Input: part model. Units: mm. Frame: model coordinates. Face numbers are marked on the shaded views. A direction names the side the tool comes from. Give positions to 0.01 mm unless a question says otherwise; leave off trailing zeros. Loops run counter-clockwise (first coordinate to the right, second up) from the corner with the lowest first, then second, coordinate; pieces in that order, holes last. Notation, with made-up numbers: (56, 54) - (87, 54) arc R18 ccw to (87, 76) - close; hole circle Ø8 at (-11, 7). An arc over 180 degrees is marked (long way). Answer as a JSON object with one key per item and string values. Group by question number.
(1) Section query D-D (x = 24.13). Return loops of the section in (y, z).
(2) Section query B-B (z = -5.08). Return loops of the section in (x, y).
(3) Mould query, pull axis Z, two halves, no side actions, for the marked faces 3, 4, 5 and 6. Classes: +Z half, -Z half, draft (parallel to the pull), parting line (faces both ways), or undercut.
(4) Section query C-C (y = 16.5). Return loops of the section in (x, z), plus the area to 3 significant figures.
(5) Section query A-A (x = 5.08). Return loops of the section in (y, z).
(6) Material intervals for L1, parallel to Z at x = 5.08, y = 2.9; L2, parallel to X at y = 2.55, z = -5.08; L3, parallel to Z at x = 24.13, y = 2.15, sorted ascending.
(7) Pin query (flat end, axial travel): P1, Ø1, axis at y = 6, z = -3, coming from the +X side; P2, Ø12, axis at y = 25, z = -22.5, coming from the -X side; P3, Ø9.5, axis at y = 23, z = -16, coming from the +X side; P4, Ø6, axis at x = 14.5, y = 25, coming from the +Z side. Return the tip coordinate at first contact, or that it passes through.
(8) Access query for the marked faces 1 and 2. Directions: +Z, -Z, +X, -X, +Y, -Y. A direction counts if a zero-diameter tool reaches every point of the face in a straight line with its end or side. Return the directions, or none.
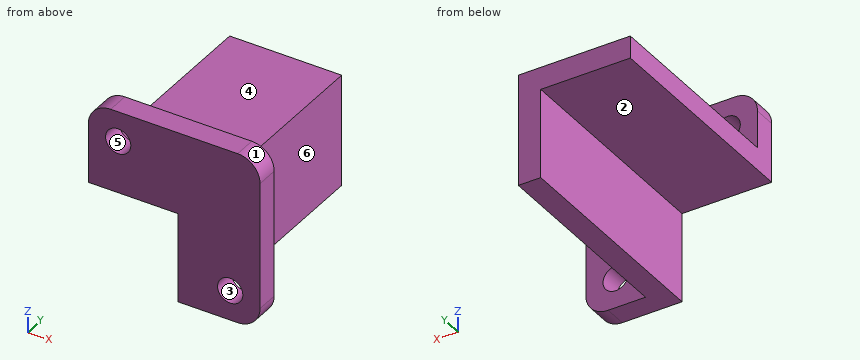
```python
from build123d import *

# Parameters (mm, degrees)
BOSS_EXTRUDE1_DEPTH = 3.81
BOSS_EXTRUDE2_DEPTH = 34.29
SKETCH3_R           = 2.15
CUT_EXTRUDE1_DEPTH  = 4.81
FILLET1_R           = 3.81


with BuildPart() as part:
    # Sketch1 → Boss-Extrude1 (new body)
    with BuildSketch(Plane(origin=(0, 0, 0), x_dir=(1, 0, 0), z_dir=(0, 1, 0))):
        Polygon((29.21, 0), (29.21, 29.21), (15.24, 29.21), (15.24, 13.97), (0, 13.97), (0, 0), align=None)
    extrude(amount=BOSS_EXTRUDE1_DEPTH)

    # Sketch2 → Boss-Extrude2 (add)
    with BuildSketch(Plane(origin=(0, 3.81, 0), x_dir=(1, 0, 0), z_dir=(0, 1, 0))):
        Polygon((0, 13.97), (15.24, 13.97), (15.24, 29.21), (19.05, 29.21), (19.05, 10.16), (0, 10.16), align=None)
    extrude(amount=BOSS_EXTRUDE2_DEPTH)

    # Sketch3 → Cut-Extrude1 (cut, through all)
    with BuildSketch(Plane(origin=(0, 3.81, 0), x_dir=(1, 0, 0), z_dir=(0, 1, 0))):
        with Locations((5.08, 5.08)):
            Circle(SKETCH3_R)
        with Locations((24.13, 24.13)):
            Circle(SKETCH3_R)
    extrude(amount=-CUT_EXTRUDE1_DEPTH, mode=Mode.SUBTRACT)

    # Fillet1
    fillet1_edges = [part.edges().sort_by_distance(p)[0] for p in [
        (29.21, 1.905, -29.21),
        (29.21, 1.905, 0),
        (0, 1.905, 0),
    ]]
    fillet(fillet1_edges, radius=FILLET1_R)


solid = part.part
```
Recorded:
{
 "1": {"outline": "(0, -29.21) - (3.81, -29.21) - (3.81, -26.28) - (0, -26.28) - close; (0, -21.98) - (3.81, -21.98) - (3.81, 0) - (0, 0) - close"},
 "2": {"outline": "(0, 0) - (2.93, 0) - (2.93, 3.81) - (0, 3.81) - close; (7.23, 0) - (29.21, 0) - (29.21, 3.81) - (7.23, 3.81) - close"},
 "3": {"face 3": "undercut", "face 4": "+Z half", "face 5": "undercut", "face 6": "draft"},
 "4": {"outline": "(0, -13.97) - (15.24, -13.97) - (15.24, -29.21) - (19.05, -29.21) - (19.05, -10.16) - (0, -10.16) - close", "area": "131 mm^2"},
 "5": {"outline": "(0, -13.97) - (38.1, -13.97) - (38.1, -10.16) - (3.81, -10.16) - (3.81, -7.23) - (0, -7.23) - close; (0, -2.93) - (3.81, -2.93) - (3.81, 0) - (0, 0) - close"},
 "6": {"L1": "z = -13.97 to -7.23, -2.93 to 0", "L2": "x = 0 to 2.93, 7.23 to 29.21", "L3": "z = -29.21 to -26.28, -21.98 to 0"},
 "7": {"P1": "passes through", "P2": "stops at x = 15.24", "P3": "stops at x = 19.05", "P4": "stops at z = -10.16"},
 "8": {"face 1": "+Z, +X, +Y, -Y", "face 2": "-Z, -X, +Y, -Y"}
}
